```python
from build123d import *

# Parameters (mm, degrees)
SKETCH1_R                 = 17.145
BOSS_EXTRUDE1_DEPTH       = 19.05
SKETCH2_R                 = 4.7625
CUT_EXTRUDE1_DEPTH        = 31.835118777
SKETCH3_R                 = 2.0193
F_10_32_TAPPED_HOLE_DEPTH = 50.8
SKETCH4_OUTSIDE_W         = 46.71
SKETCH4_OUTSIDE_H         = 46.71
SKETCH4_OUTSIDE_W_2       = 34.29
SKETCH4_OUTSIDE_H_2       = 25.4
FIT_IN_SLOT_DEPTH         = 31.83511895


with BuildPart() as part:
    # Sketch1 → Boss-Extrude1 (new body)
    with BuildSketch(Plane(origin=(0, 0, 0), x_dir=(1, 0, 0), z_dir=(0, 1, 0))):
        with Locations(Location((0, 0, 0), (0, 0, 90))):
            Circle(SKETCH1_R)
    extrude(amount=BOSS_EXTRUDE1_DEPTH)

    # Sketch2 → Cut-Extrude1 (cut, through all)
    with BuildSketch(Plane(origin=(0, 19.05, 0), x_dir=(1, 0, 0), z_dir=(0, 1, 0))):
        with Locations(Location((0, 0, 0), (0, 0, 270))):
            Circle(SKETCH2_R)
    extrude(amount=-CUT_EXTRUDE1_DEPTH, mode=Mode.SUBTRACT)

    # Sketch3 → 10-32 Tapped Hole (cut, symmetric)
    with BuildSketch(Plane.XY):
        with Locations((0, 9.525)):
            Circle(SKETCH3_R)
    extrude(amount=F_10_32_TAPPED_HOLE_DEPTH, both=True, mode=Mode.SUBTRACT)

    # Sketch4 outside → Fit in Slot (cut, through all)
    with BuildSketch(Plane(origin=(0, 19.05, 0), x_dir=(1, 0, 0), z_dir=(0, 1, 0))):
        Rectangle(SKETCH4_OUTSIDE_W, SKETCH4_OUTSIDE_H)
        Rectangle(SKETCH4_OUTSIDE_W_2, SKETCH4_OUTSIDE_H_2, mode=Mode.SUBTRACT)
    extrude(amount=-FIT_IN_SLOT_DEPTH, mode=Mode.SUBTRACT)


solid = part.part
```
Check sheet for the modelled part. Datum: model origin and axes. Units: mm. Give positions to 0.01 mm unless a question says otherwise; leave off trailing zeros. Write each loop counter-clockwise with the first axis right and the second up, starting at its lowest first coordinate (ties: lowest second). Pieces come first, ordered by that corner, then holes.
Item 1: Gauge pin test, flat ends, axial feed: pin 1 (3 mm diameter, centred on y = 16, z = 4, fed in from -X); pin 2 (3 mm diameter, centred on y = 15, z = -4, fed in from +X); pin 3 (8 mm diameter, centred on y = 8.5, z = -5.5, fed in from +X). Record the tip position at first contact, or that the pin passes through.
Item 2: Cross-section at A-A (x = 0). Enter the section's corners in (y, z).
Item 3: Draft check along X on faces 1 (the face through (-0.438, 7.554, 8.565)), 2 (the face through (0, 12, 12.7)), 3 (the face through (17.144, 9.392, 0.2)). Enter one of: released by +X, released by -X, zero draft, split by the parting line, or undercut.
Item 4: Cross-section at C-C (y = 11). Enter the section's corners in (x, z) (1 decimal).
Item 5: Cross-section at B-B (z = 1.25). Enter the section's corners in (x, y).
Item 6: Cross-section at D-D (y = 3). Enter the section's corners in (x, z) (1 decimal).
Item 7: Scan lines: L1, parallel to X at y = 11.5, z = 0 (1 decimal); L2, parallel to Z at x = 2, y = 2.75; L3, parallel to Y at x = 0, z = 5.25. Record each from-to range of solid material in increasing order.
Report:
1. pin 1: stops at x = -16.96
1. pin 2: stops at x = 16.96
1. pin 3: stops at x = 17.08
2. outline: (0, -12.7) - (7.51, -12.7) - (7.51, -4.76) - (0, -4.76) - close; (0, 4.76) - (7.51, 4.76) - (7.51, 12.7) - (0, 12.7) - close; (11.54, -12.7) - (19.05, -12.7) - (19.05, -4.76) - (11.54, -4.76) - close; (11.54, 4.76) - (19.05, 4.76) - (19.05, 12.7) - (11.54, 12.7) - close
3. face 1: undercut
3. face 2: zero draft
3. face 3: released by +X
4. outline: (-11.5, -12.7) - (-1.4, -12.7) - (-1.4, -4.6) arc R4.8 cw to (-1.4, 4.6) - (-1.4, 12.7) - (-11.5, 12.7) arc R17.1 ccw to start; (1.4, -12.7) - (11.5, -12.7) arc R17.1 ccw to (11.5, 12.7) - (1.4, 12.7) - (1.4, 4.6) arc R4.8 cw to (1.4, -4.6) - close
5. outline: (-17.1, 0) - (-4.6, 0) - (-4.6, 19.05) - (-17.1, 19.05) - close; (4.6, 0) - (17.1, 0) - (17.1, 19.05) - (4.6, 19.05) - close
6. outline: (-11.5, -12.7) - (11.5, -12.7) arc R17.1 ccw to (11.5, 12.7) - (-11.5, 12.7) arc R17.1 ccw to start; hole circle Ø9.5 at (0, 0)
7. L1: x = -17.1 to -4.8, 4.8 to 17.1
7. L2: z = -12.7 to -4.32, 4.32 to 12.7
7. L3: y = 0 to 7.51, 11.54 to 19.05
